For this review, take the finished solid that the model builds, in its own axes (mm). Face numbers are marked on the shaded views. Give positions to 0.01 mm unless a question says otherwise; leave off trailing zeros. Order: outer loops, then holes, each group sorted by start corner. A loop starts at its lowest first (then second) coordinate and runs counter-clockwise, first axis right, second up.
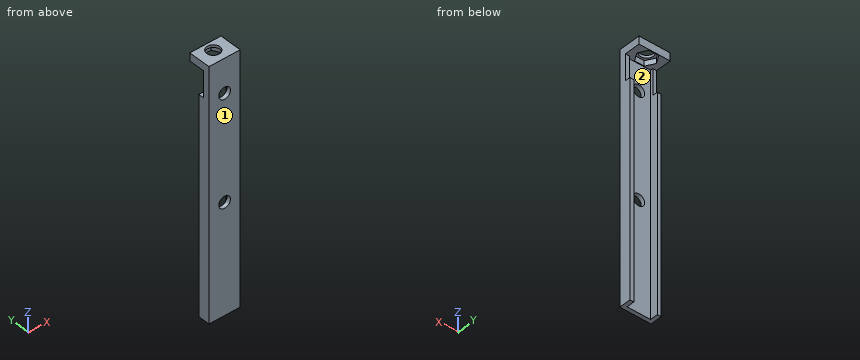
from build123d import *

# Parameters (mm, degrees)
BOSS_EXTRUDE1_DEPTH = 165
BOSS_EXTRUDE2_DEPTH = 24
BOSS_EXTRUDE3_DEPTH = 4
SKETCH3_3_R         = 5
BOSS_EXTRUDE4_DEPTH = 2
SKETCH4_R           = 4.5
CUT_EXTRUDE1_DEPTH  = 194.010362416


with BuildPart() as part:
    # Sketch1 → Boss-Extrude1 (new body)
    with BuildSketch(Plane.XY):
        Polygon((0, 0), (0, 9), (3, 9), (3, 3), (21, 3), (21, 9), (24, 9), (24, 0), align=None)
    extrude(amount=BOSS_EXTRUDE1_DEPTH)

    # Sketch2 → Boss-Extrude2 (add)
    with BuildSketch(Plane.XY.offset(165)):
        Polygon((0, 0), (24, 0), (24, 5), (21, 5), (21, 3), (3, 3), (3, 5), (0, 5), align=None)
    extrude(amount=BOSS_EXTRUDE2_DEPTH)

    # Sketch3 → Boss-Extrude3 (add)
    with BuildSketch(Plane.XY.offset(189)):
        Polygon((0, 17), (0, 5), (3, 5), (3, 3), (21, 3), (21, 5), (24, 5), (24, 17), align=None)
        Polygon((8.24722325, 16.5), (15.75277675, 16.5), (19.505553499, 10), (15.75277675, 3.5), (8.24722325, 3.5), (4.494446501, 10), align=None, mode=Mode.SUBTRACT)
    extrude(amount=-BOSS_EXTRUDE3_DEPTH)

    # Sketch3_3 → Boss-Extrude4 (add)
    # profile 1 of 3: a face of its own
    with BuildSketch(Plane.XY.offset(189)):
        Polygon((0, 17), (0, 5), (3, 5), (3, 3), (21, 3), (21, 5), (24, 5), (24, 17), align=None)
        Polygon((8.24722325, 16.5), (15.75277675, 16.5), (19.505553499, 10), (15.75277675, 3.5), (8.24722325, 3.5), (4.494446501, 10), align=None, mode=Mode.SUBTRACT)
    # profile 2 of 3: a face of its own
    with BuildSketch(Plane.XY.offset(189)):
        Polygon((3, 5), (0, 5), (0, 0), (24, 0), (24, 5), (21, 5), (21, 3), (3, 3), align=None)
    # profile 3 of 3: a face of its own
    with BuildSketch(Plane.XY.offset(189)):
        Polygon((15.75277675, 3.5), (19.505553499, 10), (15.75277675, 16.5), (8.24722325, 16.5), (4.494446501, 10), (8.24722325, 3.5), align=None)
        with Locations((12, 10)):
            Circle(SKETCH3_3_R, mode=Mode.SUBTRACT)
    extrude(amount=BOSS_EXTRUDE4_DEPTH)

    # Sketch4 → Cut-Extrude1 (cut, through all)
    with BuildSketch(Plane(origin=(0, 3, 0), x_dir=(1, 0, 0), z_dir=(0, 1, 0))):
        with Locations(Location((12, -165, 0), (0, 0, 180))):
            Circle(SKETCH4_R)
        with Locations(Location((12, -84.075, 0), (0, 0, 180))):
            Circle(SKETCH4_R)
    extrude(amount=-CUT_EXTRUDE1_DEPTH, mode=Mode.SUBTRACT)


solid = part.part
1) We need section C-C on z = 131.5. Give the boundary of the cut face in (x, y), then the cut area to 3 significant figures.
Answer sheet:
outline: (0, 0) - (24, 0) - (24, 9) - (21, 9) - (21, 3) - (3, 3) - (3, 9) - (0, 9) - close
area: 108 mm2
2) We need section B-B on y = 13.25. Give the boundary of the cut face in (x, z), then the cut area to 3 significant figures.
Answer sheet:
outline: (0, 185) - (6.37, 185) - (6.37, 189) - (8.2, 189) - (8.2, 191) - (0, 191) - close; (15.8, 189) - (17.63, 189) - (17.63, 185) - (24, 185) - (24, 191) - (15.8, 191) - close
area: 83.8 mm2
3) Clearance check with flat-ended pins moving along their axes: pin 1 (0.9 mm diameter, centred on x = 2, z = 179.5, fed in from +Y); pin 2 (9 mm diameter, centred on x = 9.5, z = 64, fed in from +Y). State where each tip first meets the part, or that it passes through.
Answer sheet:
pin 1: stops at y = 5
pin 2: stops at y = 3
4) Draft analysis for pull direction X (two halves, no side actions). For the marked faces 1 and 2, state which applies: +X half, -X half, draft (parallel to the pull), parting line (faces both ways), or undercut.
Answer sheet:
face 1: draft
face 2: undercut
5) We need section A-A on x = 12. Give the boundary of the cut face in (y, z) (3 decimals), then the cut area to 3 significant figures.
Answer sheet:
outline: (0, 0) - (3, 0) - (3, 79.575) - (0, 79.575) - close; (0, 88.575) - (3, 88.575) - (3, 160.5) - (0, 160.5) - close; (0, 169.5) - (3, 169.5) - (3, 185) - (3.5, 185) - (3.5, 189) - (5, 189) - (5, 191) - (0, 191) - close; (15, 189) - (16.5, 189) - (16.5, 185) - (17, 185) - (17, 191) - (15, 191) - close
area: 531 mm2
6) To check wall thickness, follow line 1 (Z direction, x = 12, y = 2.25) (3 decimals); line 2 (X direction, y = 5.5, z = 89.5); line 3 (Y direction, x = 12, z = 190.45). State the ranges of each line that lie inside material, in increasing order.
Answer sheet:
line 1: z = 0 to 79.575, 88.575 to 160.5, 169.5 to 191
line 2: x = 0 to 3, 21 to 24
line 3: y = 0 to 5, 15 to 17
